```python
from build123d import *

# Parameters (mm, degrees)
SKETCH1_R           = 3.25
BASE_FLANGE1_DEPTH  = 3
BOSS_EXTRUDE1_DEPTH = 30


# Sheet-metal steps are written as plain solids
with BuildPart() as part:
    # Sketch1 → Base-Flange1 (new body)
    with BuildSketch(Plane.XY):
        with BuildLine():
            Line((-79.914529915, 72.264957265), (-79.914529915, 42.264957265))
            Line((-79.914529915, 42.264957265), (-124.914529915, 42.264957265))
            ThreePointArc((-124.914529915, 42.264957265), (-128.45006382, 40.800491171), (-129.914529915, 37.264957265))
            Line((-129.914529915, 37.264957265), (-129.914529915, -152.735042735))
            ThreePointArc((-129.914529915, -152.735042735), (-128.45006382, -156.270576641), (-124.914529915, -157.735042735))
            Line((-124.914529915, -157.735042735), (65.085470085, -157.735042735))
            ThreePointArc((65.085470085, -157.735042735), (68.621003991, -156.270576641), (70.085470085, -152.735042735))
            Line((70.085470085, -152.735042735), (70.085470085, 37.264957265))
            ThreePointArc((70.085470085, 37.264957265), (68.621003991, 40.800491171), (65.085470085, 42.264957265))
            Line((65.085470085, 42.264957265), (20.085470085, 42.264957265))
            Line((20.085470085, 42.264957265), (20.085470085, 72.264957265))
            Line((20.085470085, 72.264957265), (-79.914529915, 72.264957265))
        make_face()
        with Locations((-4.914529915, 57.264957265)):
            Circle(SKETCH1_R, mode=Mode.SUBTRACT)
        with Locations((-54.914529915, 57.264957265)):
            Circle(SKETCH1_R, mode=Mode.SUBTRACT)
    extrude(amount=-BASE_FLANGE1_DEPTH)

    # Sketch2 → Boss-Extrude1 (add)
    with BuildSketch(Plane.XY):
        Polygon((42.945575149, -48.857914887), (12.945575149, -48.857914887), (12.945575149, -18.857914887), (14.945575149, -18.857914887), (14.945575149, -46.857914887), (42.945575149, -46.857914887), align=None)
        Polygon((-69.377458811, -48.857914887), (-99.377458811, -48.857914887), (-99.377458811, -78.857914887), (-97.377458811, -78.857914887), (-97.377458811, -50.857914887), (-69.377458811, -50.857914887), align=None)
    extrude(amount=BOSS_EXTRUDE1_DEPTH)


solid = part.part
```
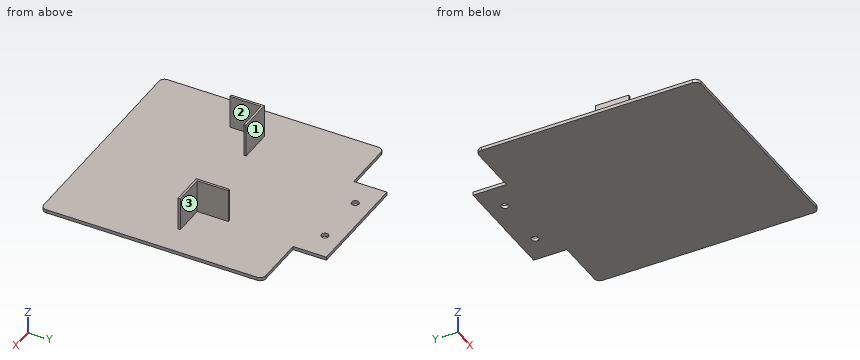
CAD build for the part. Positions are in the model's coordinates, mm. Face numbers are marked on the shaded views. A direction names the side the tool comes from. Give positions to 0.01 mm unless a question says otherwise; leave off trailing zeros. Write each loop counter-clockwise with the first axis right and the second up, starting at its lowest first coordinate (ties: lowest second). Pieces come first, ordered by that corner, then holes. Notation, with made-up numbers: M 80,38.5 L 93,38.5 A12 ccw 93,56.5 Z; hole C 15.5,60 d7. An arc over 180 degrees is marked long. Return JSON: item names as keys, results as strings. Group by question number.
(1) Drill centre lines: L1, parallel to Z at x = 20, y = -19.5; L2, parallel to Y at x = 13, z = 18; L3, parallel to Y at x = -85.5, z = 2. Where is each one in solid material? Low to high. Write a range as [from, to].
(2) Band-saw the part on C-C (x = 33.5). Give the cut face in (y, z).
(3) Band-saw the part on D-D (x = -37.5). Give the cut face in (y, z), and give its area (3 significant figures).
(4) 3-axis set-ups, long thin cutter, end or side, ignore diameter. For the marked faces 1, 2 and 3: which of +Z, -Z, +X, -X, +Y, -Y reach the whole face in a straight line?
(5) Flat gauge pins, fed straight in: pin 1 Ø10.5 at (x, y) = (-4.91, 57.26) entering from +Z; pin 2 Ø15 at (x, z) = (-91, 17.5) entering from +Y; pin 3 Ø10 at (y, z) = (-68.5, 18.5) entering from -X. Where does each tip first touch, or does it go through?
(6) Band-saw the part on A-A (z = 14). Give the cut face in (x, y), and give its area (3 significant figures).
(7) Band-saw the part on B-B (y = -42.5). Give the cut face in (x, z).
Entries:
{
 "1": {"L1": "z = [-3, 0]", "L2": "y = [-48.86, -18.86]", "L3": "y = [-50.86, -48.86]"},
 "2": {"outline": "M -157.74,-3 L 42.26,-3 L 42.26,0 L -46.86,0 L -46.86,30 L -48.86,30 L -48.86,0 L -157.74,0 Z"},
 "3": {"outline": "M -157.74,-3 L 72.26,-3 L 72.26,0 L -157.74,0 Z", "area": "690 mm^2"},
 "4": {"face 1": "+Z, -X, +Y", "face 2": "+Z, +X, -Y", "face 3": "+Z, +X, +Y"},
 "5": {"pin 1": "stops at z = 0", "pin 2": "stops at y = -48.86", "pin 3": "stops at x = -99.38"},
 "6": {"outline": "M -99.38,-78.86 L -97.38,-78.86 L -97.38,-50.86 L -69.38,-50.86 L -69.38,-48.86 L -99.38,-48.86 Z; M 12.95,-48.86 L 42.95,-48.86 L 42.95,-46.86 L 14.95,-46.86 L 14.95,-18.86 L 12.95,-18.86 Z", "area": "232 mm^2"},
 "7": {"outline": "M -129.91,-3 L 70.09,-3 L 70.09,0 L 14.95,0 L 14.95,30 L 12.95,30 L 12.95,0 L -129.91,0 Z"}
}
